Input: part model. Units: mm. Frame: model coordinates. A direction names the side the tool comes from. Coordinates: 2 decimals unless noted, no trailing zeros. Loops run counter-clockwise (first coordinate to the right, second up) from the corner with the lowest first, then second, coordinate; pieces in that order, holes last. Notation, with made-up numbers: (20.5, 29) - (41.5, 29) arc R17 cw to (41.5, 33) - close; hole circle Ø3 at (14.5, 62.5). An arc over 180 degrees is marked (long way). Answer as CSV lines item,"result". Start each with the question number.
```python
from build123d import *

# Parameters (mm, degrees)
SKETCH_3_W               = 97.5
SKETCH_3_H               = 27
EXTRUDE_1_DEPTH          = 3
SKETCH_4_R               = 1.25
CUT_EXTRUDE_1_DEPTH      = 51.673587795
SKETCH_7_W               = 4
SKETCH_7_H               = 8
EXTRUDE_2_DEPTH          = 5
SKETCH_8_W               = 38
SKETCH_8_H               = 9
EXTRUDE_3_DEPTH          = 3
FILLET_3_R               = 8
FILLET_4_R               = 2
CUT_EXTRUDE_4_DEPTH      = 55.284551355
CUT_EXTRUDE_4_DEPTH_BACK = 5
SKETCH_9_W               = 4
SKETCH_9_H               = 8
SKETCH_13_R              = 1.5
CUT_EXTRUDE_7_DEPTH      = 54.775575449
SKETCH_16_R              = 3
CUT_EXTRUDE_9_DEPTH      = 2
CUT_EXTRUDE_10_DEPTH     = 10
FILLET_5_R               = 8
FILLET_6_R               = 2
HOLE_WIZARD_M3_1_D       = 2.5
HOLE_WIZARD_M3_1_DEPTH   = 3
HOLE_WIZARD_M3_1_TIP     = 0.751075774


with BuildPart() as part:
    # 草图3 → 凸台-拉伸1 (new body)
    with BuildSketch(Plane.XY):
        Rectangle(SKETCH_3_W, SKETCH_3_H)
    extrude(amount=EXTRUDE_1_DEPTH)

    # 草图4 → 切除-拉伸1 (cut, through all)
    with BuildSketch(Plane.XY.offset(3)):
        with Locations((-43.25, 11)):
            Circle(SKETCH_4_R)
        with Locations((-43.25, -11)):
            Circle(SKETCH_4_R)
        with Locations((31.75, 11)):
            Circle(SKETCH_4_R)
        with Locations((31.75, -11)):
            Circle(SKETCH_4_R)
        with Locations((17.25, 11)):
            Circle(SKETCH_4_R)
        with Locations((-12.75, 11)):
            Circle(SKETCH_4_R)
    extrude(amount=-CUT_EXTRUDE_1_DEPTH, mode=Mode.SUBTRACT)

    # 草图7 → 凸台-拉伸2 (add)
    with BuildSketch(Plane(origin=(0, 0, 0), x_dir=(-1, 0, 0), z_dir=(0, 0, -1))):
        with Locations((46.75, 0.5)):
            Rectangle(SKETCH_7_W, SKETCH_7_H)
        with Locations((-46.75, 0.5)):
            Rectangle(SKETCH_7_W, SKETCH_7_H)
    extrude(amount=EXTRUDE_2_DEPTH)

    # 草图8 → 凸台-拉伸3 (add)
    with BuildSketch(Plane.XY.offset(3)):
        with Locations((3.25, 18)):
            Rectangle(SKETCH_8_W, SKETCH_8_H)
        with BuildLine():
            Line((-11.75, 20.5), (18.25, 20.5))
            ThreePointArc((18.25, 20.5), (20.25, 18.5), (18.25, 16.5))
            Line((18.25, 16.5), (-11.75, 16.5))
            ThreePointArc((-11.75, 16.5), (-13.75, 18.5), (-11.75, 20.5))
        make_face(mode=Mode.SUBTRACT)
    extrude(amount=-EXTRUDE_3_DEPTH)

    # 圆角3
    fillet_3_edges = [part.edges().sort_by_distance(p)[0] for p in [
        (22.25, 13.5, 1.5),
        (-15.75, 13.5, 1.5),
    ]]
    fillet(fillet_3_edges, radius=FILLET_3_R)

    # 圆角4
    fillet_4_edges = [part.edges().sort_by_distance(p)[0] for p in [
        (-15.75, 22.5, 1.5),
        (22.25, 22.5, 1.5),
    ]]
    fillet(fillet_4_edges, radius=FILLET_4_R)

    # 草图9 → 切除-拉伸4 (cut, two sides: drawn at the far end of the back side and taken through both)
    with BuildSketch(Plane(origin=(0, 0, -5), x_dir=(-1, 0, 0), z_dir=(0, 0, -1)).offset(-CUT_EXTRUDE_4_DEPTH_BACK)):
        with Locations((-46.75, 0.5)):
            Rectangle(SKETCH_9_W, SKETCH_9_H)
        with Locations((46.75, 0.5)):
            Rectangle(SKETCH_9_W, SKETCH_9_H)
    extrude(amount=CUT_EXTRUDE_4_DEPTH + CUT_EXTRUDE_4_DEPTH_BACK, mode=Mode.SUBTRACT)

    # 草图13 → 切除-拉伸7 (cut, through all)
    with BuildSketch(Plane(origin=(0, 0, 0), x_dir=(-1, 0, 0), z_dir=(0, 0, -1))):
        with Locations((-43.75, 0)):
            Circle(SKETCH_13_R)
        with Locations((43.75, 0)):
            Circle(SKETCH_13_R)
    extrude(amount=-CUT_EXTRUDE_7_DEPTH, mode=Mode.SUBTRACT)

    # 草图16 → 切除-拉伸9 (cut)
    with BuildSketch(Plane.XY.offset(3)):
        with Locations((-43.75, 0)):
            Circle(SKETCH_16_R)
        with Locations((43.75, 0)):
            Circle(SKETCH_16_R)
    extrude(amount=-CUT_EXTRUDE_9_DEPTH, mode=Mode.SUBTRACT)

    # 草图17 → 切除-拉伸10 (cut)
    with BuildSketch(Plane(origin=(0, 0, 0), x_dir=(-1, 0, 0), z_dir=(0, 0, -1))):
        Polygon((39.25, -8), (39.25, 8), (-27.75, 8), (-29.75, 8), (-29.75, -9.826666667), (-27.75, -9.826666667), (39.25, -9.826666667), align=None)
    extrude(amount=-CUT_EXTRUDE_10_DEPTH, mode=Mode.SUBTRACT)

    # 圆角5
    fillet_5_edges = [part.edges().sort_by_distance(p)[0] for p in [
        (29.75, 8, 1.5),
        (-39.25, 8, 1.5),
        (-39.25, -9.826666667, 1.5),
        (29.75, -9.826666667, 1.5),
    ]]
    fillet(fillet_5_edges, radius=FILLET_5_R)

    # 圆角6
    fillet_6_edges = [part.edges().sort_by_distance(p)[0] for p in [
        (48.75, -13.5, 1.5),
        (-48.75, -13.5, 1.5),
        (-48.75, 13.5, 1.5),
        (48.75, 13.5, 1.5),
    ]]
    fillet(fillet_6_edges, radius=FILLET_6_R)

    # M3 螺纹孔1
    with Locations(Plane(origin=(-43.25, 11, 3), x_dir=(1, 0, 0), z_dir=(0, 0, 1))):
        with Locations((0, 0), (0, -22), (30.5, 0), (60.5, 0), (75, 0), (75, -22)):
            Hole(HOLE_WIZARD_M3_1_D / 2, depth=HOLE_WIZARD_M3_1_DEPTH)
            with Locations((0, 0, -(HOLE_WIZARD_M3_1_DEPTH + HOLE_WIZARD_M3_1_TIP / 2))):  # 118° drill point
                Cone(0, HOLE_WIZARD_M3_1_D / 2, HOLE_WIZARD_M3_1_TIP, mode=Mode.SUBTRACT)


solid = part.part
```
Item 1: Set-up query: faces 5 (the flat face through (38, 13.5, 1)), 6 (the cylindrical face through (-46.747, 0.132, 2.014)), 7 (the flat face through (-1, -13.5, 1)), 8 (the flat face through (3, 20.5, 2)), 9 (the cylindrical face through (-48.15, -12.93, 1.52)). Return all of +Z, -Z, +X, -X, +Y, -Y with unobstructed straight access to the full face (end or side cutting, diameter ignored); none if empty.
Item 2: Section query C-C, the plane x = 31.75. Output: boundary loops of the cut face in (y, z).
Item 3: Section query A-A, the plane x = 43.75. Output: boundary loops of the cut face in (y, z), and give its area (3 significant figures).
Item 4: Draft query along X for faces 1 (the flat face through (-42, -1, 1)), 2 (the flat face through (48.75, 0, 1)), 3 (the cylindrical face through (-36.844, 5.719, 1.521)), 4 (the cylindrical face through (-18.445, 15.512, 1.479)). Return one class per face: pulls with the +X half, pulls with the -X half, needs draft (parallel to the pull), parting line crosses it, or undercut.
Item 5: Material intervals for probe 1 along Y at (x, z) = (31.75, 2.05); probe 2 along Y at (x, z) = (17.25, 2.35); probe 3 along Y at (x, z) = (11.5, 1.05), sorted ascending.
Item 6: Section query D-D, the plane x = -12.75. Output: boundary loops of the cut face in (y, z).
Item 7: Contact query for flat-ended pins moving along their axis: P1, Ø2, axis at x = 17.25, y = 11, coming from the +Z side; P2, Ø0.9, axis at x = -15, z = 2, coming from the +Y side; P3, Ø3, axis at x = 43.5, y = -1, coming from the +Z side. Output: stop coordinate, or through.
Item 8: Section query B-B, the plane y = -5.5. Output: boundary loops of the cut face in (x, z), and give its area (3 significant figures).
Response values:
1,face 5,"+Z, -Z, +X, +Y"
1,face 6,"+Z"
1,face 7,"+Z, -Z, +X, -X, -Y"
1,face 8,"+Z, -Z"
1,face 9,"+Z, -Z, -X, -Y"
2,outline,"(-13.5, 0) - (-12.25, 0) - (-12.25, 3) - (-13.5, 3) - close; (-9.75, 0) - (9.75, 0) - (9.75, 3) - (-9.75, 3) - close; (12.25, 0) - (13.5, 0) - (13.5, 3) - (12.25, 3) - close"
3,outline,"(-13.5, 0) - (-1.5, 0) - (-1.5, 1) - (-3, 1) - (-3, 3) - (-13.5, 3) - close; (1.5, 0) - (13.5, 0) - (13.5, 3) - (3, 3) - (3, 1) - (1.5, 1) - close"
3,area,"66.0 mm²"
4,face 1,"undercut"
4,face 2,"pulls with the +X half"
4,face 3,"undercut"
4,face 4,"pulls with the -X half"
5,probe 1,"y = -13.5 to -12.25, -9.75 to 9.75, 12.25 to 13.5"
5,probe 2,"y = -13.5 to -9.83, 8 to 9.75, 12.25 to 16.5, 20.5 to 22.5"
5,probe 3,"y = -13.5 to -9.83, 8 to 16.5, 20.5 to 22.5"
6,outline,"(-13.5, 0) - (-9.83, 0) - (-9.83, 3) - (-13.5, 3) - close; (8, 0) - (9.75, 0) - (9.75, 3) - (8, 3) - close; (12.25, 0) - (16.77, 0) - (16.77, 3) - (12.25, 3) - close; (20.23, 0) - (22.5, 0) - (22.5, 3) - (20.23, 3) - close"
7,P1,"passes through"
7,P2,"stops at y = 22.35"
7,P3,"stops at z = 1"
8,outline,"(-48.75, 0) - (-38.36, 0) - (-38.36, 3) - (-48.75, 3) - close; (28.86, 0) - (48.75, 0) - (48.75, 3) - (28.86, 3) - close"
8,area,"90.9 mm²"
